Design review of the part built by this model. Coordinates are the model's own, in mm. A direction names the side the tool comes from. Coordinates: 2 decimals unless noted, no trailing zeros. Loops run counter-clockwise (first coordinate to the right, second up) from the corner with the lowest first, then second, coordinate; pieces in that order, holes last. Notation, with made-up numbers: (-38.75, 34.5) - (-25.75, 34.5) arc R11 cw to (-25.75, 53.5) - close; hole circle Ø8 at (-25, 47). An arc over 180 degrees is marked (long way). Use one line per item in the form item = value. Start each with the question number.
(1) Tool access review of faces 4 (the face through (0, 129, 1159.675)), 5 (the face through (396, 0, -0.005)), 6 (the face through (370, 0, 49.995)), 7 (the face through (361, 229.8, 1185)), 8 (the face through (20, -25, 557)): name each direction out of +Z, -Z, +X, -X, +Y, -Y from which nothing blocks a thin tool from reaching the whole face with its end or side.
(2) Clearance check with a flat-ended pin moving along its axis: pin 1 Ø8 at (y, z) = (226.5, 556.5) entering from -X. State where the tip first meets the part, or that it passes through.
(3) The part is to be moulded in two halves that separate along X. For faces 1 (the face through (-25, 14, 608)), 2 (the face through (0, 229.8, 613)), 3 (the face through (314, 25, 25)), say which applies: pulls with the +X half, pulls with the -X half, needs draft (parallel to the pull), parting line crosses it, or undercut.
(4) Add section A-A (x = 420.5). State the section outline as (y, z) points (3 decimals), plus the area to 4 significant figures.
(5) Add section B-B (y = 253.5). State the section outline as (x, z) points (3 decimals).
(6) For L1, parallel to Z at x = 682.5, y = 0 (3 decimals); L2, parallel to X at y = 246, z = 718; L3, parallel to Y at x = 10.5, z = 758.5, list the stretches that pass through material, from the lowest coordinate up.
(7) Add section C-C (z = 1008.5). State the section outline as (x, y) points, plus the area to 3 significant figures.
```python
from build123d import *

# Parameters (mm, degrees)
SKETCH2_W            = 50
SKETCH2_H            = 50
BOSS_EXTRUDE1_DEPTH  = 1209.675
SKETCH3_W            = 50
SKETCH3_H            = 50
BOSS_EXTRUDE2_DEPTH  = 731.05
SKETCH4_W            = 50
SKETCH4_H            = 50
BOSS_EXTRUDE3_DEPTH  = 1159.68
SKETCH6_W            = 50
SKETCH6_H            = 50
BOSS_EXTRUDE4_DEPTH  = 681.05
SKETCH8_W            = 50
SKETCH8_H            = 50
BOSS_EXTRUDE5_DEPTH  = 254.8
SKETCH9_W            = 50
SKETCH9_H            = 50
BOSS_EXTRUDE6_DEPTH  = 731.05
SKETCH10_W           = 50
SKETCH10_H           = 50
BOSS_EXTRUDE7_DEPTH  = 204.8
SKETCH11_W           = 50
SKETCH11_H           = 49.995
BOSS_EXTRUDE8_DEPTH  = 254.8
SKETCH12_W           = 50
SKETCH12_H           = 50
BOSS_EXTRUDE9_DEPTH  = 1109.8
SKETCH13_W           = 50
SKETCH13_H           = 50
BOSS_EXTRUDE10_DEPTH = 1109.8
SKETCH14_W           = 50
SKETCH14_H           = 49.995
BOSS_EXTRUDE11_DEPTH = 254.8
SKETCH15_W           = 49.995
SKETCH15_H           = 50
BOSS_EXTRUDE12_DEPTH = 681.05


with BuildPart() as part:
    # Sketch2 → Boss-Extrude1 (new body)
    with BuildSketch(Plane.XY):
        Rectangle(SKETCH2_W, SKETCH2_H)
    extrude(amount=BOSS_EXTRUDE1_DEPTH)

    # Sketch3 → Boss-Extrude2 (add)
    with BuildSketch(Plane(origin=(25, 0, 0), x_dir=(0, 0, -1), z_dir=(1, 0, 0))):
        with Locations((-1184.675, 0)):
            Rectangle(SKETCH3_W, SKETCH3_H)
    extrude(amount=BOSS_EXTRUDE2_DEPTH)

    # Sketch4 → Boss-Extrude3 (add)
    with BuildSketch(Plane(origin=(0, 0, 1159.675), x_dir=(-1, 0, 0), z_dir=(0, 0, -1))):
        with Locations((-731.05, 0)):
            Rectangle(SKETCH4_W, SKETCH4_H)
    extrude(amount=BOSS_EXTRUDE3_DEPTH)

    # Sketch6 → Boss-Extrude4 (add)
    with BuildSketch(Plane.ZY.offset(-706.05)):
        with Locations((24.995, 0)):
            Rectangle(SKETCH6_W, SKETCH6_H)
    extrude(amount=BOSS_EXTRUDE4_DEPTH)

    # Sketch8 → Boss-Extrude5 (add)
    with BuildSketch(Plane(origin=(0, 25, 0), x_dir=(1, 0, 0), z_dir=(0, 1, 0))):
        with Locations((0, -1184.675)):
            Rectangle(SKETCH8_W, SKETCH8_H)
    extrude(amount=BOSS_EXTRUDE5_DEPTH)

    # Sketch9 → Boss-Extrude6 (add)
    with BuildSketch(Plane(origin=(25, 0, 0), x_dir=(0, 0, -1), z_dir=(1, 0, 0))):
        with Locations((-1184.675, 254.8)):
            Rectangle(SKETCH9_W, SKETCH9_H)
    extrude(amount=BOSS_EXTRUDE6_DEPTH)

    # Sketch10 → Boss-Extrude7 (add)
    with BuildSketch(Plane.XZ.offset(-229.8)):
        with Locations((731.05, 1184.675)):
            Rectangle(SKETCH10_W, SKETCH10_H)
    extrude(amount=BOSS_EXTRUDE7_DEPTH)

    # Sketch11 → Boss-Extrude8 (add)
    with BuildSketch(Plane(origin=(0, 25, 0), x_dir=(1, 0, 0), z_dir=(0, 1, 0))):
        with Locations((731.05, -24.9975)):
            Rectangle(SKETCH11_W, SKETCH11_H)
    extrude(amount=BOSS_EXTRUDE8_DEPTH)

    # Sketch12 → Boss-Extrude9 (add)
    with BuildSketch(Plane(origin=(0, 0, 1159.675), x_dir=(-1, 0, 0), z_dir=(0, 0, -1))):
        with Locations((-731.05, 254.8)):
            Rectangle(SKETCH12_W, SKETCH12_H)
    extrude(amount=BOSS_EXTRUDE9_DEPTH)

    # Sketch13 → Boss-Extrude10 (add)
    with BuildSketch(Plane(origin=(0, 0, 1159.675), x_dir=(-1, 0, 0), z_dir=(0, 0, -1))):
        with Locations((0, 254.8)):
            Rectangle(SKETCH13_W, SKETCH13_H)
    extrude(amount=BOSS_EXTRUDE10_DEPTH)

    # Sketch14 → Boss-Extrude11 (add)
    with BuildSketch(Plane(origin=(0, 25, 0), x_dir=(1, 0, 0), z_dir=(0, 1, 0))):
        with Locations((0, -24.9975)):
            Rectangle(SKETCH14_W, SKETCH14_H)
    extrude(amount=BOSS_EXTRUDE11_DEPTH)

    # Sketch15 → Boss-Extrude12 (add)
    with BuildSketch(Plane(origin=(25, 0, 0), x_dir=(0, 0, -1), z_dir=(1, 0, 0))):
        with Locations((-24.9975, 254.8)):
            Rectangle(SKETCH15_W, SKETCH15_H)
    extrude(amount=BOSS_EXTRUDE12_DEPTH)


solid = part.part
```
Computed values:
q1.face_4 = +X, -X
q1.face_5 = -Z, +X, -X, +Y, -Y
q1.face_6 = +Y, -Y
q1.face_7 = +Z, -Z
q1.face_8 = +Z, -Z, +X, -X, -Y
q2.pin_1 = -25
q3.face_1 = pulls with the -X half
q3.face_2 = needs draft
q3.face_3 = undercut
q4.outline = (-25, -0.005) - (25, -0.005) - (25, 49.995) - (-25, 49.995) - close; (-25, 1159.675) - (25, 1159.675) - (25, 1209.675) - (-25, 1209.675) - close; (229.8, 0) - (279.8, 0) - (279.8, 49.995) - (229.8, 49.995) - close; (229.8, 1159.675) - (279.8, 1159.675) - (279.8, 1209.675) - (229.8, 1209.675) - close
q4.area = 10,000 mm^2
q5.outline = (-25, 0) - (756.05, 0) - (756.05, 1209.675) - (-25, 1209.675) - close; hole (25, 49.995) - (706.05, 49.995) - (706.05, 1159.675) - (25, 1159.675) - close
q6.L1 = -0.005 to 49.995, 1159.675 to 1209.675
q6.L2 = -25 to 25, 706.05 to 756.05
q6.L3 = -25 to 25, 229.8 to 279.8
q7.outline = (-25, -25) - (25, -25) - (25, 25) - (-25, 25) - close; (-25, 229.8) - (25, 229.8) - (25, 279.8) - (-25, 279.8) - close; (706.05, -25) - (756.05, -25) - (756.05, 25) - (706.05, 25) - close; (706.05, 229.8) - (756.05, 229.8) - (756.05, 279.8) - (706.05, 279.8) - close
q7.area = 10,000 mm^2
